from build123d import *

# Parameters (mm, degrees)
BOSS_EXTRUDE1_DEPTH = 11
SKETCH2_W           = 3.5
SKETCH2_H           = 32
BOSS_EXTRUDE2_DEPTH = 50
SKETCH3_R           = 10.25
SKETCH3_R_2         = 1.783609491
SKETCH3_R_3         = 1.426196869
CUT_EXTRUDE1_DEPTH  = 50
SKETCH4_R           = 2.22645949
CUT_EXTRUDE2_DEPTH  = 36
SKETCH5_R           = 1.95657882
CUT_EXTRUDE3_DEPTH  = 32


with BuildPart() as part:
    # Sketch1 → Boss-Extrude1 (new body)
    with BuildSketch(Plane(origin=(0, 0, 0), x_dir=(1, 0, 0), z_dir=(0, 1, 0))):
        with BuildLine():
            Line((38, 16), (0, 16))
            Line((0, 16), (0, 7.5))
            ThreePointArc((0, 7.5), (5.303300859, 5.303300859), (7.5, 0))
            ThreePointArc((7.5, 0), (5.303300859, -5.303300859), (0, -7.5))
            Line((0, -7.5), (0, -16))
            Line((0, -16), (38, -16))
            Line((38, -16), (38, 16))
        make_face()
    boss_extrude1 = extrude(amount=BOSS_EXTRUDE1_DEPTH)

    # Sketch2 → Boss-Extrude2 (add)
    with BuildSketch(Plane(origin=(0, 11, 0), x_dir=(1, 0, 0), z_dir=(0, 1, 0))):
        with Locations((36.25, 0)):
            Rectangle(SKETCH2_W, SKETCH2_H)
    boss_extrude2 = extrude(amount=BOSS_EXTRUDE2_DEPTH)

    # Sketch3 → Cut-Extrude1 (cut)
    with BuildSketch(Plane.ZY.offset(-34.5)):
        with Locations((0, 23)):
            Circle(SKETCH3_R)
        with Locations((-11, 17.202811543)):
            Circle(SKETCH3_R_2)
        with Locations((11, 17.202811543)):
            Circle(SKETCH3_R_3)
    cut_extrude1 = extrude(amount=-CUT_EXTRUDE1_DEPTH, mode=Mode.SUBTRACT)

    # Sketch4 → Cut-Extrude2 (cut)
    with BuildSketch(Plane(origin=(0, 0, -16), x_dir=(-1, 0, 0), z_dir=(0, 0, -1))):
        with Locations((-15, 5.5)):
            Circle(SKETCH4_R)
    cut_extrude2 = extrude(amount=-CUT_EXTRUDE2_DEPTH, mode=Mode.SUBTRACT)

    # Mirror1: Boss-Extrude1, Boss-Extrude2, Cut-Extrude1, Cut-Extrude2 across plane
    add(boss_extrude1.mirror(Plane(origin=(0, 11, 0), x_dir=(0, 0, 1), z_dir=(1, 0, 0))))
    add(boss_extrude2.mirror(Plane(origin=(0, 11, 0), x_dir=(0, 0, 1), z_dir=(1, 0, 0))))
    add(cut_extrude1.mirror(Plane(origin=(0, 11, 0), x_dir=(0, 0, 1), z_dir=(1, 0, 0))), mode=Mode.SUBTRACT)
    add(cut_extrude2.mirror(Plane(origin=(0, 11, 0), x_dir=(0, 0, 1), z_dir=(1, 0, 0))), mode=Mode.SUBTRACT)

    # Sketch5 → Cut-Extrude3 (cut)
    with BuildSketch(Plane.XY.offset(16)):
        with Locations((0, 5)):
            Circle(SKETCH5_R)
    extrude(amount=-CUT_EXTRUDE3_DEPTH, mode=Mode.SUBTRACT)


solid = part.part
Verification items for the finished model (mm, model axes). A direction names the side the tool comes from. Give positions to 0.01 mm unless a question says otherwise; leave off trailing zeros. Write each loop counter-clockwise with the first axis right and the second up, starting at its lowest first coordinate (ties: lowest second). Pieces come first, ordered by that corner, then holes.
(1) Material ranges on line 1 (X direction, y = 26, z = -14); line 2 (Y direction, x = 36.5, z = 11); line 3 (Y direction, x = 0, z = 8), recorded low to high.
(2) Cross-section at C-C (z = -6). Enter the section's corners in (x, y).
(3) Gauge pin test, flat ends, axial feed: pin 1 (4.5 mm diameter, centred on y = 17.2, z = 11, fed in from -X); pin 2 (18.5 mm diameter, centred on y = 23, z = 0, fed in from +X); pin 3 (4 mm diameter, centred on x = 4.5, z = 3.5, fed in from +Y). Record the tip position at first contact, or that the pin passes through.
(4) Cross-section at B-B (y = 10). Enter the section's corners in (x, z), plus the area to 3 significant figures.
(5) Mould release check, pull along X, two halves, no side actions. Record for faces 3 (the face through (36.23, 18.97, -11.23)), 4 (the face through (-0.25, 6.94, 11.68)), 5 (the face through (38, 37, 0)): +X half, -X half, draft (parallel to the pull), parting line (faces both ways), or undercut.
(6) Cross-section at A-A (x = 15). Enter the section's corners in (y, z), plus the area to 3 significant figures.
(7) Access from +Z, -Z, +X, -X, +Y, -Y to the whole of each face (thin tool, end or side, straight path). Record for faces 1 (the face through (-36.226, 12.994, -2.222)), 2 (the face through (-34.5, 41, 0)).
(8) Cross-section at D-D (y = 54). Enter the section's corners in (x, z), plus the area to 3 significant figures.
Worked out:
1. line 1: x = -38 to -34.5, 34.5 to 38
1. line 2: y = 0 to 15.78, 18.63 to 61
1. line 3: y = 0 to 3.04, 6.96 to 11
2. outline: (-38, 0) - (-4.5, 0) - (-4.5, 11) - (-34.5, 11) - (-34.5, 14.69) - (-38, 14.69) - close; (-38, 31.31) - (-34.5, 31.31) - (-34.5, 61) - (-38, 61) - close; (4.5, 0) - (38, 0) - (38, 14.69) - (34.5, 14.69) - (34.5, 11) - (4.5, 11) - close; (34.5, 31.31) - (38, 31.31) - (38, 61) - (34.5, 61) - close; hole circle Ø4.45 at (-15, 5.5); hole circle Ø4.45 at (15, 5.5)
3. pin 1: stops at x = -38
3. pin 2: passes through
3. pin 3: stops at y = 11
4. outline: (-38, -16) - (38, -16) - (38, 16) - (-38, 16) - close; hole circle Ø15 at (0, 0)
4. area: 2,260 mm2
5. face 3: draft
5. face 4: undercut
5. face 5: +X half
6. outline: (0, -16) - (3.27, -16) - (3.27, 16) - (0, 16) - close; (7.73, -16) - (11, -16) - (11, 16) - (7.73, 16) - close
6. area: 210 mm2
7. face 1: +X, -X
7. face 2: +Z, -Z, +Y
8. outline: (-38, -16) - (-34.5, -16) - (-34.5, 16) - (-38, 16) - close; (34.5, -16) - (38, -16) - (38, 16) - (34.5, 16) - close
8. area: 224 mm2
